Design review of the part built by this model. Coordinates are the model's own, in mm. A direction names the side the tool comes from. Give positions to 0.01 mm unless a question says otherwise; leave off trailing zeros. Order: outer loops, then holes, each group sorted by start corner. A loop starts at its lowest first (then second) coordinate and runs counter-clockwise, first axis right, second up. Notation, with made-up numbers: M -23.5,-2 L -5.5,-2 A20 cw -5.5,22 Z; hole C -37.5,74 d4. An arc over 180 degrees is marked long. Answer as a JSON object with one key per item and string values.
from build123d import *

# Parameters (mm, degrees)
SKETCH1_W           = 7
SKETCH1_H           = 4.5
BOSS_EXTRUDE1_DEPTH = 5.83
SKETCH2_R           = 2.15
BOSS_EXTRUDE2_DEPTH = 1.6
SKETCH3_R           = 2
BOSS_EXTRUDE3_DEPTH = 3.8
SKETCH4_R           = 0.445
BOSS_EXTRUDE4_DEPTH = 3.3


with BuildPart() as part:
    # Sketch1 → Boss-Extrude1 (new body)
    with BuildSketch(Plane(origin=(0, 0, 0), x_dir=(1, 0, 0), z_dir=(0, 1, 0))):
        with Locations((3.5, -2.25)):
            Rectangle(SKETCH1_W, SKETCH1_H)
    extrude(amount=BOSS_EXTRUDE1_DEPTH)

    # Sketch2 → Boss-Extrude2 (add)
    with BuildSketch(Plane(origin=(0, 5.83, 0), x_dir=(1, 0, 0), z_dir=(0, 1, 0))):
        with Locations((3.5, -2.25)):
            Circle(SKETCH2_R)
    extrude(amount=BOSS_EXTRUDE2_DEPTH)

    # Sketch3 → Boss-Extrude3 (add)
    with BuildSketch(Plane(origin=(0, 7.43, 0), x_dir=(1, 0, 0), z_dir=(0, 1, 0))):
        with Locations((3.5, -2.25)):
            Circle(SKETCH3_R)
    extrude(amount=BOSS_EXTRUDE3_DEPTH)

    # Sketch4 → Boss-Extrude4 (add)
    with BuildSketch(Plane.XZ):
        with Locations((1, 3.7)):
            Circle(SKETCH4_R)
        with Locations((3.54, 3.7)):
            Circle(SKETCH4_R)
        with Locations((6.08, 3.7)):
            Circle(SKETCH4_R)
        with Locations((6.08, 1.16)):
            Circle(SKETCH4_R)
        with Locations((3.54, 1.16)):
            Circle(SKETCH4_R)
        with Locations((1, 1.16)):
            Circle(SKETCH4_R)
    extrude(amount=BOSS_EXTRUDE4_DEPTH)


solid = part.part
(1) Draft analysis for pull direction Z (two halves, no side actions). For faces 4 (the cylindrical face through (5.635, -1.627, 1.18)), 5 (the flat face through (6, -3.3, 1)), 6 (the cylindrical face through (1.41, -1.63, 3.53)), 7 (the flat face through (3, 3, 4.5)), state which applies: +Z half, -Z half, draft (parallel to the pull), parting line (faces both ways), or undercut.
Checked values:
{"face 4": "undercut", "face 5": "draft", "face 6": "undercut", "face 7": "+Z half"}
(2) We need section A-A (x = 6.08). Write out the cut boundary in (y, z) (3 decimals), plus the area to 3 significant figures.
Checked values:
{"outline": "M -3.3,0.715 L 0,0.715 L 0,0 L 5.83,0 L 5.83,4.5 L 0,4.5 L 0,4.145 L -3.3,4.145 L -3.3,3.255 L 0,3.255 L 0,1.605 L -3.3,1.605 Z", "area": "32.1 mm^2"}
(3) We need section C-C (y = 8.25). Write out the cut boundary in (x, z).
Checked values:
{"outline": "C 3.5,2.25 d4"}
(4) Tool access review of faces 1 (the flat face through (1, -3.3, 3.7)), 2 (the flat face through (3, 0, 2)), 3 (the cylindrical face through (1.913, 9.303, 3.467)): name each direction out of +Z, -Z, +X, -X, +Y, -Y from which nothing blocks a thin tool from reaching the whole face with its end or side.
Checked values:
{"face 1": "+Z, -Z, +X, -X, -Y", "face 2": "-Y", "face 3": "+Y"}
(5) We need section D-D (z = 1.45). Write out the cut boundary in (x, y), plus the area to 3 significant figures.
Checked values:
{"outline": "M 0,0 L 0.66,0 L 0.66,-3.3 L 1.34,-3.3 L 1.34,0 L 3.2,0 L 3.2,-3.3 L 3.88,-3.3 L 3.88,0 L 5.74,0 L 5.74,-3.3 L 6.42,-3.3 L 6.42,0 L 7,0 L 7,5.83 L 5.5,5.83 L 5.5,7.43 L 5.33,7.43 L 5.33,11.23 L 1.67,11.23 L 1.67,7.43 L 1.5,7.43 L 1.5,5.83 L 0,5.83 Z", "area": "67.8 mm^2"}
(6) To check wall thickness, follow L1, parallel to Z at x = 1, y = -0.5 (3 decimals); L2, parallel to Y at x = 3.75, z = 0.6; L3, parallel to Y at x = 6.75, z = 2.1. State the ranges of each line that lie inside material, in increasing order. Write a range as from..to.
Checked values:
{"L1": "z = 0.715..1.605, 3.255..4.145", "L2": "y = 0..11.23", "L3": "y = 0..5.83"}
